Work out the finished part from the listing and answer in its coordinate system (mm). A direction names the side the tool comes from. Coordinates: 2 decimals unless noted, no trailing zeros. Order: outer loops, then holes, each group sorted by start corner. A loop starts at its lowest first (then second) coordinate and runs counter-clockwise, first axis right, second up. Notation, with made-up numbers: M 25.5,-1 L 53.5,-1 A35 ccw 53.5,33 Z; hole C 43,89.5 d4. An arc over 180 degrees is marked long. Use a Markdown table: item, result.
Autodesk Inventor part; units mm, degrees
ref_plane "YZ Plane" through (0, 0, 0) normal (1, 0, 0) x (0, 1, 0)
ref_plane "XZ Plane" through (0, 0, 0) normal (0, 1, 0) x (-1, 0, 0)
ref_plane "XY Plane" through (0, 0, 0) normal (0, 0, 1) x (1, 0, 0)
sketch "Esboço1" plane through (0, 0, 0) normal (0, 1, 0) x (-1, 0, 0)
  line L0 (0, 0) -> (15, 0)
  line L1 (15, 0) -> (15, -15)
  line L2 (15, -15) -> (0, -15)
  line L3 (0, -15) -> (0, 0)
  dimension "d0" = 15
  dimension "d1" = 15
extrude "Extrusão1" add sketch "Esboço1" along normal blind 20
sketch "Esboço2" plane through (0, 0, 0) normal (1, 0, 0) x (0, 0, -1)
  point P0 (0, 0)
  point P1 (7.5, 7.5)
hole "Furo1" at (0, 7.5, -7.5) direction (-1, 0, 0) diameter 8 depth 12
sketch "Esboço4" plane through (0, 20, 0) normal (0, 1, 0) x (1, 0, 0)
  point P0 (0, 0)
  point P1 (-7.5, 7.5)
hole "Furo2" at (-7.5, 20, -7.5) direction (0, -1, 0) diameter 8 depth 7.5
fillet "Arredondamento1" radius 2 12 edges at (-7.5, 20, 0) (-15, 10, 0) (-15, 20, -7.5) (-7.5, 0, 0) (-15, 0, -7.5) (-15, 10, -15) (-7.5, 0, -15) (-7.5, 20, -15) (0, 10, -15) (0, 0, -7.5) (0, 10, 0) (0, 20, -7.5)
properties part number "cantoneira"
1. For a pull along Z with two mould halves and no side action, classify faces 3 (the face through (-12, 7, -7)), 4 (the face through (-8, 12.5, -8)), 5 (the face through (-14.4, 0.57, -7.58)), 6 (the face through (-0.6, 10.11, -0.57)) as +Z half, -Z half, draft (parallel to the pull), parting line (faces both ways), or undercut.
Answers below:
| item | result |
|---|---|
| face 3 | undercut |
| face 4 | undercut |
| face 5 | draft |
| face 6 | +Z half |
2. Section B-B on y = 14.25 is taken. Determine the outline of the cut face in (x, z).
Answers below:
| item | result |
|---|---|
| outline | M -15,-13 A2 ccw -13,-15 L -2,-15 A2 ccw 0,-13 L 0,-2 A2 ccw -2,0 L -13,0 A2 ccw -15,-2 Z; hole C -7.5,-7.5 d8 |
3. Section A-A on x = -3 is taken. Determine the outline of the cut face in (y, z), then the cut area to 3 significant figures.
Answers below:
| item | result |
|---|---|
| outline | M 0,-13 A2 ccw 2,-15 L 18,-15 A2 ccw 20,-13 L 20,-2 A2 ccw 18,0 L 2,0 A2 ccw 0,-2 Z; hole C 7.5,-7.5 d8 |
| area | 246 mm² |
4. Section C-C on z = -7.5 is taken. Determine the outline of the cut face in (x, y).
Answers below:
| item | result |
|---|---|
| outline | M -15,2 A2 ccw -13,0 L -2,0 A2 ccw 0,2 L 0,3.5 L -12,3.5 L -12,11.5 L 0,11.5 L 0,18 A2 ccw -2,20 L -3.5,20 L -3.5,12.5 L -11.5,12.5 L -11.5,20 L -13,20 A2 ccw -15,18 Z |
5. Section D-D on y = 2.5 is taken. Determine the outline of the cut face in (x, z).
Answers below:
| item | result |
|---|---|
| outline | M -15,-13 A2 ccw -13,-15 L -2,-15 A2 ccw 0,-13 L 0,-2 A2 ccw -2,0 L -13,0 A2 ccw -15,-2 Z |
6. For faces 1 (the face through (-7.58, 0.57, -0.6)), 2 (the face through (-6.084, 7.324, -3.504)), determine the directions among +Z, -Z, +X, -X, +Y, -Y from which every point of the face is accessible in a straight line to the end or side of a thin tool.
Answers below:
| item | result |
|---|---|
| face 1 | +Z, +X, -X, -Y |
| face 2 | +X |
7. Find the intervals of material crossed by probe 1 along Y at (x, z) = (-6.75, -7.5); probe 2 along X at (y, z) = (15, -7.5), in increasing order.
Answers below:
| item | result |
|---|---|
| probe 1 | 0 to 3.5, 11.5 to 12.5 |
| probe 2 | -15 to -11.5, -3.5 to 0 |
